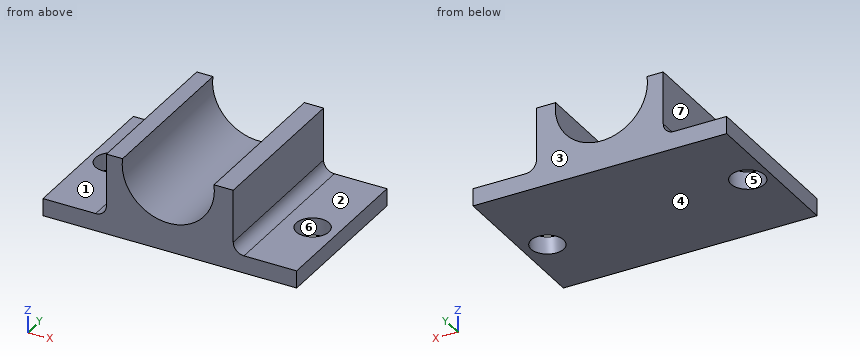
from build123d import *

# Parameters (mm, degrees)
F1_DEPTH = 76.2
F2_R     = 5.08
F3_R     = 7.707036
F3_R_2   = 7.889442
F4_DEPTH = 25.4


with BuildPart() as f1:
    # F0 (on Front) → F1 (new body)
    with BuildSketch(Plane.XZ):
        with BuildLine():
            Line((-63.861191, -13.506276), (-63.861191, -21.727486))
            Line((-63.861191, -21.727486), (55.933593, -21.727486))
            Line((55.933593, -21.727486), (55.933593, -13.506276))
            Line((55.933593, -13.506276), (25.984896, -13.506276))
            Line((25.984896, -13.506276), (25.984896, 16.442422))
            Line((25.984896, 16.442422), (16.882844, 16.442422))
            ThreePointArc((16.882844, 16.442422), (-4.697835, -8.147052), (-26.278514, 16.442422))
            Line((-26.278514, 16.442422), (-33.912495, 16.442422))
            Line((-33.912495, 16.442422), (-33.912495, -13.506276))
            Line((-33.912495, -13.506276), (-63.861191, -13.506276))
        make_face()
    extrude(amount=F1_DEPTH)

    # F2
    f2_edges = [f1.edges().sort_by_distance(p)[0] for p in [
        (-33.912495, -38.1, -13.506276),
        (25.984896, -38.1, -13.506276),
    ]]
    fillet(f2_edges, radius=F2_R)

    # F3 (on face) → F4 (cut)
    with BuildSketch(Plane.XY.offset(-13.506276)):
        with Locations((44.482626, -42.280514)):
            Circle(F3_R)
        with Locations((-53.291064, -36.701836)):
            Circle(F3_R_2)
    extrude(amount=-F4_DEPTH, mode=Mode.SUBTRACT)


solid = f1.part
Can you work these out from the model? Positions are in its coordinate system, mm. Face numbers are marked on the shaded views. A direction names the side the tool comes from. Round coordinates to 2 decimals unless told otherwise and drop trailing zeros. Order: outer loops, then holes, each group sorted by start corner. A loop starts at its lowest first (then second) coordinate and runs counter-clockwise, first axis right, second up. Notation, with made-up numbers: M -29.75,38.25 L 23.25,38.25 A21 cw 23.25,68.25 Z; hole C -10,3 d11. An arc over 180 degrees is marked long. Use a Markdown table: item, result.
1) Imagine slicing it at D-D (y = -12). List the corners of the cut face in (x, z) for me, then the cut area to 3 significant figures.
Geometry says:
| item | result |
|---|---|
| outline | M -63.86,-21.73 L 55.93,-21.73 L 55.93,-13.51 L 31.06,-13.51 A5.08 cw 25.98,-8.43 L 25.98,16.44 L 16.88,16.44 A21.76 cw long -26.28,16.44 L -33.91,16.44 L -33.91,-8.43 A5.08 cw -38.99,-13.51 L -63.86,-13.51 Z |
| area | 1,920 mm² |
2) Imagine slicing it at A-A (z = 9). List the corners of the cut face in (x, y) for me, then the cut area to 3 significant figures.
Geometry says:
| item | result |
|---|---|
| outline | M -33.91,-76.2 L -25.97,-76.2 L -25.97,0 L -33.91,0 Z; M 16.57,-76.2 L 25.98,-76.2 L 25.98,0 L 16.57,0 Z |
| area | 1,320 mm² |
3) On a 3-axis mill with a long thin cutter (end or side, diameter ignored), from which of +Z, -Z, +X, -X, +Y, -Y can I reach the whole of each face in a straight line? I mean the marked faces 1, 2 and 3. Say none if no direction works.
Geometry says:
| item | result |
|---|---|
| face 1 | +Z, -X, +Y, -Y |
| face 2 | +Z, +X, +Y, -Y |
| face 3 | +Z, -Z, +X, -X, +Y |
4) If we mould it in two halves opening along X, with no side actions, what happens to the marked faces 4, 5, 6 and 7? For each: +X half, -X half, draft (parallel to the pull), parting line (faces both ways), or undercut.
Geometry says:
| item | result |
|---|---|
| face 4 | draft |
| face 5 | undercut |
| face 6 | undercut |
| face 7 | -X half |
5) I'm going to push flat-ended pins straight in: P1, Ø6, axis at x = -5, y = -35, coming from the +Z side; P2, Ø2, axis at y = -50, z = 12, coming from the +X side; P3, Ø7.5, axis at x = -56, y = -33, coming from the +Z side; P4, Ø20, axis at x = 44.48, y = -42.28, coming from the -Z side. Where does each tip first touch, or does it pass through?
Geometry says:
| item | result |
|---|---|
| P1 | stops at z = -7.9 |
| P2 | stops at x = 25.98 |
| P3 | stops at z = -13.51 |
| P4 | stops at z = -21.73 |
6) Imagine slicing it at B-B (y = -46). List the corners of the cut face in (x, z) for me, then the cut area to 3 significant figures.
Geometry says:
| item | result |
|---|---|
| outline | M -63.86,-21.73 L 37.73,-21.73 L 37.73,-13.51 L 31.06,-13.51 A5.08 cw 25.98,-8.43 L 25.98,16.44 L 16.88,16.44 A21.76 cw long -26.28,16.44 L -33.91,16.44 L -33.91,-8.43 A5.08 cw -38.99,-13.51 L -63.86,-13.51 Z; M 51.23,-21.73 L 55.93,-21.73 L 55.93,-13.51 L 51.23,-13.51 Z |
| area | 1,810 mm² |
7) If I drill on line 1 along X through (y, z) = (-42, -19); line 2 along X through (y, z) = (-71, 14); line 3 along Z through (x, y) = (-52.5, -17.5), over which ranges is the centre line in solid material (lowest first)?
Geometry says:
| item | result |
|---|---|
| line 1 | x = -63.86 to -59.14, -47.45 to 36.78, 52.18 to 55.93 |
| line 2 | x = -33.91 to -26.46, 17.06 to 25.98 |
| line 3 | z = -21.73 to -13.51 |
8) Imagine slicing it at C-C (x = -52.5). List the corners of the cut face in (y, z) for me.
Geometry says:
| item | result |
|---|---|
| outline | M -76.2,-21.73 L -44.55,-21.73 L -44.55,-13.51 L -76.2,-13.51 Z; M -28.85,-21.73 L 0,-21.73 L 0,-13.51 L -28.85,-13.51 Z |
